Check sheet for the modelled part. Datum: model origin and axes. Units: mm. A direction names the side the tool comes from. Round coordinates to 2 decimals unless told otherwise and drop trailing zeros. Write each loop counter-clockwise with the first axis right and the second up, starting at its lowest first coordinate (ties: lowest second). Pieces come first, ordered by that corner, then holes.
Item 1: Cross-section at B-B on y = 5.7. Enter the section's corners in (x, z), plus the area to 3 significant figures.
Item 2: Cross-section at C-C on z = 0. Enter the section's corners in (x, y).
Item 3: Material ranges on line 1 (Y direction, x = 5.25, z = -18); line 2 (X direction, y = 7, z = 3); line 3 (X direction, y = 1.55, z = -10.85), recorded low to high.
Item 4: Go/stop test with flat-tipped pins: pin 1 Ø1 at (x, z) = (-9, -7) entering from +Y; pin 2 Ø7.5 at (x, z) = (1.5, -3) entering from +Y. Record where each tip stops, or that it passes through.
Item 5: Release check for a two-part mould opening along Z. For faces 1 (the flat face through (0, 3.5, 5)), 2 (the flat face through (-5, 4.2, -18)), 3 (the cylindrical face through (11.3, 5.07, 18.32)) record: +Z half, -Z half, draft (parallel to the pull), parting line (faces both ways), or undercut.
Item 6: Cross-section at D-D on x = 1.25. Enter the section's corners in (y, z).
Item 7: Tool access check on faces 4 (the cylindrical face through (11.01, 7.89, 0.12)), 5 (the flat face through (0, 1.5, 13)), 6 (the flat face through (-9.75, 6, -18)). Record the directions out of +Z, -Z, +X, -X, +Y, -Y that give a thin tool (end or side, any length) a straight path to the whole face; none if there is none.
Item 8: Cross-section at A-A on x = -2.5. Enter the section's corners in (y, z).
from build123d import *

# Parameters (mm, degrees)
SKETCH_2_W          = 23.5
SKETCH_2_H          = 37.5
EXTRUDE_1_DEPTH     = 10
SHELL_1_T           = -1.5
FILLET_1_R          = 1.5
SKETCH_3_W          = 20.5
SKETCH_3_H          = 25.5
EXTRUDE_2_DEPTH     = 2
SKETCH_4_W          = 20.5
SKETCH_4_H          = 10
CUT_EXTRUDE_1_DEPTH = 2
FILLET_2_R          = 1.5
SKETCH_6_W          = 10
SKETCH_6_H          = 4
CUT_EXTRUDE_2_DEPTH = 2
SKETCH_7_R          = 1.5
CUT_EXTRUDE_3_DEPTH = 2
SKETCH_8_R          = 0.9
CUT_EXTRUDE_4_DEPTH = 3
SKETCH_9_R          = 0.9
CUT_EXTRUDE_5_DEPTH = 3


with BuildPart() as part:
    # 草图2 → 凸台-拉伸1 (new body)
    with BuildSketch(Plane(origin=(0, 0, 0), x_dir=(1, 0, 0), z_dir=(0, 1, 0))):
        Rectangle(SKETCH_2_W, SKETCH_2_H)
    extrude(amount=EXTRUDE_1_DEPTH)

    # 抽壳1
    shell_1_openings = [part.faces().sort_by_distance(p)[0] for p in [
        (0, 10, 0),
    ]]
    offset(amount=SHELL_1_T, openings=shell_1_openings, kind=Kind.INTERSECTION)

    # 圆角1
    fillet_1_edges = [part.edges().sort_by_distance(p)[0] for p in [
        (-11.75, 5, -18.75),
        (11.75, 5, -18.75),
        (11.75, 5, 18.75),
        (-11.75, 5, 18.75),
    ]]
    fillet(fillet_1_edges, radius=FILLET_1_R)

    # 草图3 → 凸台-拉伸2 (add)
    with BuildSketch(Plane(origin=(0, 1.5, 0), x_dir=(1, 0, 0), z_dir=(0, 1, 0))):
        with Locations((0, 4.5)):
            Rectangle(SKETCH_3_W, SKETCH_3_H)
    extrude(amount=EXTRUDE_2_DEPTH)

    # 草图4 → 切除-拉伸1 (cut)
    with BuildSketch(Plane(origin=(0, 3.5, 0), x_dir=(1, 0, 0), z_dir=(0, 1, 0))):
        with Locations((0, 2.25)):
            Rectangle(SKETCH_4_W, SKETCH_4_H)
    extrude(amount=-CUT_EXTRUDE_1_DEPTH, mode=Mode.SUBTRACT)

    # 圆角2
    fillet_2_edges = [part.edges().sort_by_distance(p)[0] for p in [
        (0, 1.5, -7.25),
        (0, 1.5, 2.75),
    ]]
    fillet(fillet_2_edges, radius=FILLET_2_R)

    # 草图6 → 切除-拉伸2 (cut)
    with BuildSketch(Plane(origin=(0, 0, -18.75), x_dir=(-1, 0, 0), z_dir=(0, 0, -1))):
        with Locations((4.75, 6.2)):
            Rectangle(SKETCH_6_W, SKETCH_6_H)
    extrude(amount=-CUT_EXTRUDE_2_DEPTH, mode=Mode.SUBTRACT)

    # 草图7 → 切除-拉伸3 (cut)
    with BuildSketch(Plane(origin=(0, 0, -18.75), x_dir=(-1, 0, 0), z_dir=(0, 0, -1))):
        with Locations((-5.25, 5.7)):
            Circle(SKETCH_7_R)
    extrude(amount=-CUT_EXTRUDE_3_DEPTH, mode=Mode.SUBTRACT)

    # 草图8 → 切除-拉伸4 (cut)
    with BuildSketch(Plane(origin=(0, 3.5, 0), x_dir=(1, 0, 0), z_dir=(0, 1, 0))):
        with Locations(Location((7.85, 10.85, 0), (0, 0, 270))):
            Circle(SKETCH_8_R)
    extrude(amount=-CUT_EXTRUDE_4_DEPTH, mode=Mode.SUBTRACT)

    # 草图9 → 切除-拉伸5 (cut)
    with BuildSketch(Plane(origin=(11.75, 0, 0), x_dir=(0, 0, -1), z_dir=(1, 0, 0))):
        with Locations((0, 7)):
            Circle(SKETCH_9_R)
    extrude(amount=-CUT_EXTRUDE_5_DEPTH, mode=Mode.SUBTRACT)


solid = part.part
Response values:
1. outline: (-11.75, -17.25) arc R1.5 ccw to (-10.25, -18.75) - (-9.75, -18.75) - (-9.75, -17.25) - (-10.25, -17.25) - (-10.25, 17.25) - (10.25, 17.25) - (10.25, -17.25) - (6.75, -17.25) - (6.75, -18.75) - (10.25, -18.75) arc R1.5 ccw to (11.75, -17.25) - (11.75, 17.25) arc R1.5 ccw to (10.25, 18.75) - (-10.25, 18.75) arc R1.5 ccw to (-11.75, 17.25) - close; (0.25, -18.75) - (3.75, -18.75) - (3.75, -17.25) - (0.25, -17.25) - close
1. area: 153 mm2
2. outline: (-11.75, 0) - (11.75, 0) - (11.75, 6.1) - (10.25, 6.1) - (10.25, 1.5) - (-10.25, 1.5) - (-10.25, 10) - (-11.75, 10) - close; (10.25, 7.9) - (11.75, 7.9) - (11.75, 10) - (10.25, 10) - close
3. line 1: y = 0 to 4.2, 7.2 to 10
3. line 2: x = -11.75 to -10.25, 10.25 to 11.75
3. line 3: x = -11.75 to 6.95, 8.75 to 11.75
4. pin 1: stops at y = 3.5
4. pin 2: stops at y = 1.88
5. face 1: undercut
5. face 2: draft
5. face 3: +Z half
6. outline: (0, -18.75) - (10, -18.75) - (10, -17.25) - (3.5, -17.25) - (3.5, -7.25) - (3, -7.25) arc R1.5 cw to (1.5, -5.75) - (1.5, 1.25) arc R1.5 cw to (3, 2.75) - (3.5, 2.75) - (3.5, 8.25) - (1.5, 8.25) - (1.5, 17.25) - (10, 17.25) - (10, 18.75) - (0, 18.75) - close
7. face 4: +X
7. face 5: +Y
7. face 6: -Z
8. outline: (0, -18.75) - (4.2, -18.75) - (4.2, -17.25) - (3.5, -17.25) - (3.5, -7.25) - (3, -7.25) arc R1.5 cw to (1.5, -5.75) - (1.5, 1.25) arc R1.5 cw to (3, 2.75) - (3.5, 2.75) - (3.5, 8.25) - (1.5, 8.25) - (1.5, 17.25) - (10, 17.25) - (10, 18.75) - (0, 18.75) - close; (8.2, -18.75) - (10, -18.75) - (10, -17.25) - (8.2, -17.25) - close
